from build123d import *

# Parameters (mm, degrees)
F0_R     = 1.5
F0_W     = 10
F0_H     = 10
F1_DEPTH = 3
F2_SIZE  = 1
F3_SIZE  = 5


with BuildPart() as f1:
    # F0 (on Top) → F1 (new body)
    with BuildSketch(Plane.XY):
        with BuildLine():
            Line((95.505033, 15), (74.505033, 15))
            ThreePointArc((74.505033, 15), (-76, 0), (74.505033, -15))
            Line((74.505033, -15), (95.505033, -15))
            Line((95.505033, -15), (95.505033, 0))
            Line((95.505033, 0), (95.505033, 15))
        make_face()
        with Locations((0, -73)):
            Circle(F0_R, mode=Mode.SUBTRACT)
        with Locations((-73, 0)):
            Circle(F0_R, mode=Mode.SUBTRACT)
        with BuildLine():
            ThreePointArc((69.8212, 5), (69.955286, 2.501598), (70, 0))
            ThreePointArc((70, 0), (69.955286, -2.501598), (69.8212, -5))
            ThreePointArc((69.8212, -5), (-70, 0), (69.8212, 5))
        make_face(mode=Mode.SUBTRACT)
        with Locations((0, 73)):
            Circle(F0_R, mode=Mode.SUBTRACT)
        with Locations((73, 0)):
            Circle(F0_R, mode=Mode.SUBTRACT)
        with Locations((84.505033, 0)):
            Rectangle(F0_W, F0_H, mode=Mode.SUBTRACT)
    extrude(amount=F1_DEPTH)

    # F2
    f2_edges = [f1.edges().sort_by_distance(p)[0] for p in [
        (-76, 0, 0),
        (-69.8212, -5, 0),
    ]]
    chamfer(f2_edges, length=F2_SIZE)

    # F3
    f3_edges = [f1.edges().sort_by_distance(p)[0] for p in [
        (95.505033, -15, 1.5),
        (95.505033, 15, 1.5),
    ]]
    chamfer(f3_edges, length=F3_SIZE)


solid = f1.part
Read the model definition and answer for the solid it produces. Units are mm, in the model's axes. Round coordinates to 2 decimals unless told otherwise and drop trailing zeros. Loops run counter-clockwise (first coordinate to the right, second up) from the corner with the lowest first, then second, coordinate; pieces in that order, holes last.
Q1. Section A-A on z = 1.6 is taken. Write down the section's boundary in (x, y).
Q2. Each of these flat-tipped pins is pushed along its axis until it touches: pin 1 (1.5 mm diameter, centred on x = -14, z = 2.5, fed in from +Y); pin 2 (0.9 mm diameter, centred on x = 79, z = 1, fed in from -Y); pin 3 (2.5 mm diameter, centred on x = 73, y = 0, fed in from +Z). Where does it stop, or does it pass through?
Q3. Determine the mould class of faces 1 (the face through (-69.935, -3.008, 1.986)), 2 (the face through (73, -5, 0)), 3 (the face through (-75.096, 3.096, 0.16)) for opening direction Y: released by +Y, released by -Y, zero draft, split by the parting line, or undercut.
Q4. Consider probe 1 along Y at (x, z) = (0, 1.95); probe 2 along X at (y, z) = (-0.5, 1.7); probe 3 along Y at (x, z) = (0, 0.95). Determine where each line is inside the solid, lowest interval first.
Output:
1. outline: (74.51, -15) - (90.51, -15) - (95.51, -10) - (95.51, 10) - (90.51, 15) - (74.51, 15) arc R76 ccw (long way) to start; hole circle Ø3 at (-73, 0); hole circle Ø3 at (0, -73); hole circle Ø3 at (0, 73); hole (69.82, -5) arc R70 ccw to (70, 0) arc R70 ccw to (69.82, 5) arc R70 ccw (long way) to start; hole circle Ø3 at (73, 0); hole (79.51, -5) - (89.51, -5) - (89.51, 5) - (79.51, 5) - close
2. pin 1: stops at y = 74.84
2. pin 2: stops at y = -15
2. pin 3: passes through
3. face 1: undercut
3. face 2: zero draft
3. face 3: split by the parting line
4. probe 1: y = -76 to -74.5, -71.5 to -70, 70 to 71.5, 74.5 to 76
4. probe 2: x = -76 to -74.41, -71.59 to -70, 70 to 71.59, 74.41 to 79.51, 89.51 to 95.51
4. probe 3: y = -75.95 to -74.5, -71.5 to -70.05, 70.05 to 71.5, 74.5 to 75.95
